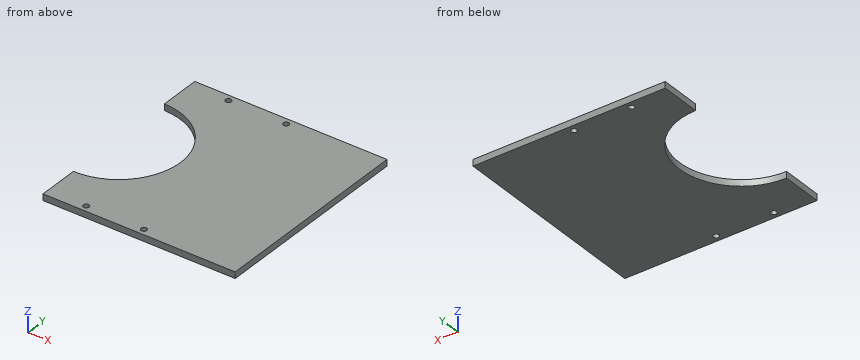
```python
from build123d import *

# Parameters (mm, degrees)
BOSS_EXTRUDE1_DEPTH     = 5
CUT_EXTRUDE1_DEPTH      = 110.772492001
CUT_EXTRUDE1_DEPTH_BACK = 110.772492001
SKETCH2_R               = 2.25


with BuildPart() as part:
    # Sketch1 → Boss-Extrude1 (new body)
    with BuildSketch(Plane(origin=(0, 0, 0), x_dir=(0, 1, 0), z_dir=(0, 0, 1))):
        with BuildLine():
            Line((-48, 75), (-80, 75))
            Line((-80, 75), (-80, -75))
            Line((-80, -75), (80, -75))
            Line((80, -75), (80, 75))
            Line((80, 75), (48, 75))
            ThreePointArc((48, 75), (0, 27), (-48, 75))
        make_face()
    extrude(amount=BOSS_EXTRUDE1_DEPTH)

    # Sketch2 → Cut-Extrude1 (cut, two sides: drawn at the far end of the back side and taken through both)
    with BuildSketch(Plane.XY.offset(5).offset(-CUT_EXTRUDE1_DEPTH_BACK)):
        with Locations((0, -75)):
            Circle(SKETCH2_R)
        with Locations((-45, -75)):
            Circle(SKETCH2_R)
        with Locations((0, 75)):
            Circle(SKETCH2_R)
        with Locations((-45, 75)):
            Circle(SKETCH2_R)
    extrude(amount=CUT_EXTRUDE1_DEPTH + CUT_EXTRUDE1_DEPTH_BACK, mode=Mode.SUBTRACT)


solid = part.part
```
Geometry check sheet. Reference: the model listing, model coordinates, mm. Coordinates: 2 decimals unless noted, no trailing zeros. Order: outer loops, then holes, each group sorted by start corner. A loop starts at its lowest first (then second) coordinate and runs counter-clockwise, first axis right, second up. Notation, with made-up numbers: (51, -13) - (95, -13) arc R7 cw to (95, -5) - close; hole circle Ø2 at (-19.75, 1.25). An arc over 180 degrees is marked (long way). Use one line per item in the form item = value.
1. Section check D-D (x = -45). Record the boundary of the cut face in (y, z), then the cut area to 3 significant figures.
Here are the results:
outline = (-80, 0) - (-77.25, 0) - (-77.25, 5) - (-80, 5) - close; (-72.75, 0) - (-37.47, 0) - (-37.47, 5) - (-72.75, 5) - close; (37.47, 0) - (72.75, 0) - (72.75, 5) - (37.47, 5) - close; (77.25, 0) - (80, 0) - (80, 5) - (77.25, 5) - close
area = 380 mm²
2. Scan lines: line 1 (X direction, y = 75, z = 2.55); line 2 (Y direction, x = 0, z = 1.5); line 3 (Y direction, x = -45, z = 2.8). Record each from-to range of solid material in increasing order.
Here are the results:
line_1 = -75 to -47.25, -42.75 to -2.25, 2.25 to 75
line_2 = -80 to -77.25, -72.75 to 72.75, 77.25 to 80
line_3 = -80 to -77.25, -72.75 to -37.47, 37.47 to 72.75, 77.25 to 80
3. Section check B-B (y = 75). Record the boundary of the cut face in (x, z).
Here are the results:
outline = (-75, 0) - (-47.25, 0) - (-47.25, 5) - (-75, 5) - close; (-42.75, 0) - (-2.25, 0) - (-2.25, 5) - (-42.75, 5) - close; (2.25, 0) - (75, 0) - (75, 5) - (2.25, 5) - close
4. Section check C-C (z = 3.3). Record the boundary of the cut face in (x, y).
Here are the results:
outline = (-75, -80) - (75, -80) - (75, 80) - (-75, 80) - (-75, 48) arc R48 cw to (-75, -48) - close; hole circle Ø4.5 at (-45, -75); hole circle Ø4.5 at (-45, 75); hole circle Ø4.5 at (0, -75); hole circle Ø4.5 at (0, 75)
5. Section check A-A (x = 0). Record the boundary of the cut face in (y, z).
Here are the results:
outline = (-80, 0) - (-77.25, 0) - (-77.25, 5) - (-80, 5) - close; (-72.75, 0) - (72.75, 0) - (72.75, 5) - (-72.75, 5) - close; (77.25, 0) - (80, 0) - (80, 5) - (77.25, 5) - close
